from build123d import *

# Parameters (mm, degrees)
BOSS_EXTRUDE1_DEPTH = 3.175
SKETCH2_R           = 3.175
CUT_EXTRUDE1_DEPTH  = 4.175


with BuildPart() as part:
    # Sketch1 → Boss-Extrude1 (new body)
    with BuildSketch(Plane(origin=(0, 0, 0), x_dir=(0, 0, -1), z_dir=(1, 0, 0))):
        with BuildLine():
            Line((-50.8, 0), (-50.8, -25.4))
            Line((-50.8, -25.4), (-25.4, -12.7))
            Line((-25.4, -12.7), (-25.4, 0))
            ThreePointArc((-25.4, 0), (0, 25.4), (25.4, 0))
            Line((25.4, 0), (25.4, -50.8))
            ThreePointArc((25.4, -50.8), (22.983175157, -62.950198978), (16.100640303, -73.250640303))
            Line((16.100640303, -73.250640303), (3.130634922, -86.220645683))
            ThreePointArc((3.130634922, -86.220645683), (-3.886063261, -96.721876619), (-6.35, -109.108923092))
            Line((-6.35, -109.108923092), (19.05, -109.108923092))
            ThreePointArc((19.05, -109.108923092), (19.580476865, -106.442035801), (21.091147164, -104.181157925))
            Line((21.091147164, -104.181157925), (34.061152545, -91.211152545))
            ThreePointArc((34.061152545, -91.211152545), (46.449715283, -72.67035816), (50.8, -50.8))
            Line((50.8, -50.8), (50.8, 0))
            ThreePointArc((50.8, 0), (0, 50.8), (-50.8, 0))
        make_face()
    extrude(amount=BOSS_EXTRUDE1_DEPTH)

    # Sketch2 → Cut-Extrude1 (cut, through all)
    with BuildSketch(Plane(origin=(3.175, 0, 0), x_dir=(0, 0, -1), z_dir=(1, 0, 0))):
        with Locations((38.1, 0)):
            Circle(SKETCH2_R)
        with Locations((-32.995567884, 19.05)):
            Circle(SKETCH2_R)
        with Locations((34.71644522, -67.810278569)):
            Circle(SKETCH2_R)
        with Locations((6.35, -102.758923092)):
            Circle(SKETCH2_R)
    extrude(amount=-CUT_EXTRUDE1_DEPTH, mode=Mode.SUBTRACT)


solid = part.part
The model under review builds one solid part; all positions refer to its coordinate system, in mm. A direction names the side the tool comes from. Coordinates: 2 decimals unless noted, no trailing zeros. Loops run counter-clockwise (first coordinate to the right, second up) from the corner with the lowest first, then second, coordinate; pieces in that order, holes last.
(1) Consider section C-C, the plane x = 1.9. Give the boundary of the cut face in (y, z) (3 decimals).
Determined:
outline: (-109.109, -19.05) arc R6.969 cw to (-104.181, -21.091) - (-91.211, -34.061) arc R57.15 ccw to (-50.8, -50.8) - (0, -50.8) arc R50.8 ccw to (0, 50.8) - (-25.4, 50.8) - (-12.7, 25.4) - (0, 25.4) arc R25.4 cw to (0, -25.4) - (-50.8, -25.4) arc R31.75 cw to (-73.251, -16.101) - (-86.221, -3.131) arc R32.369 ccw to (-109.109, 6.35) - close; hole circle Ø6.35 at (-102.759, -6.35); hole circle Ø6.35 at (-67.81, -34.716); hole circle Ø6.35 at (0, -38.1); hole circle Ø6.35 at (19.05, 32.996)
(2) Consider section D-D, the plane y = -46. Give the boundary of the cut face in (x, z) (3 decimals), plus the area to 3 significant figures.
Determined:
outline: (0, -50.8) - (3.175, -50.8) - (3.175, -25.4) - (0, -25.4) - close
area: 80.6 mm2
(3) Wall thickness on L1, parallel to Y at x = 2.8, z = -35.5; L2, parallel to Z at x = 1, y = 1.5; L3, parallel to Y at x = 1.6, z = -4.5: over which ranges is each line inside the solid? List them lowest first.
Determined:
L1: y = -89.72 to -70.89, -64.73 to -1.82, 1.82 to 36.34
L2: z = -50.78 to -40.9, -35.3 to -25.36, 25.36 to 50.78
L3: y = -109.11 to -105.34, -100.18 to -84.85, 25 to 50.6
(4) Consider section A-A, the plane y = -7.5. Give the boundary of the cut face in (x, z) (3 decimals).
Determined:
outline: (0, -50.8) - (3.175, -50.8) - (3.175, -25.4) - (0, -25.4) - close; (0, 25.4) - (3.175, 25.4) - (3.175, 50.8) - (0, 50.8) - close
(5) Tool access review of faces 1 (the cylindrical face through (1.565, 25.394, 0.559)), 2 (the cylindrical face through (1.565, 50.788, -1.117)), 3 (the flat face through (2, -19, 38)), 4 (the flat face through (0, -10, -33)), 5 (the flat face through (1.57, -79.64, -9.71)): name each direction out of +Z, -Z, +X, -X, +Y, -Y from which nothing blocks a thin tool from reaching the whole face with its end or side.
Determined:
face 1: +X, -X
face 2: +X, -X, +Y
face 3: +X, -X, -Y
face 4: +Z, -Z, -X, +Y, -Y
face 5: +Z, +X, -X
(6) Draft analysis for pull direction Y (two halves, no side actions). For faces 6 (the cylindrical face through (1.61, -65.66, -32.38)), 7 (the cylindrical face through (1.6, 17.1, 35.5)), 8 (the cylindrical face through (1.565, -106.477, -19.566)), 9 (the flat face through (3.175, -10, -33)), state which applies: +Y half, -Y half, draft (parallel to the pull), parting line (faces both ways), or undercut.
Determined:
face 6: undercut
face 7: undercut
face 8: -Y half
face 9: draft
(7) Insertion check: P1, Ø5, axis at y = 19.05, z = 33, coming from the -X side; P2, Ø1, axis at x = 2, z = -2.5, coming from the +Y side; P3, Ø1, axis at x = 1, y = -33.5, coming from the +Z side; P4, Ø7.5, axis at y = -67.81, z = -34.72, coming from the -X side. Each pin has a flat end and moves straight along its axis. Give the tip position at first contact, or say it passes through.
Determined:
P1: passes through
P2: stops at y = 50.76
P3: stops at z = -25.4
P4: stops at x = 0
(8) Consider section B-B, the plane z = 0. Give the boundary of the cut face in (x, y) (3 decimals), plus the area to 3 significant figures.
Determined:
outline: (0, -109.109) - (3.175, -109.109) - (3.175, -89.854) - (0, -89.854) - close; (0, 25.4) - (3.175, 25.4) - (3.175, 50.8) - (0, 50.8) - close
area: 142 mm2
